from build123d import *

# Parameters (mm, degrees)
BOSS_EXTRUDE1_DEPTH            = 300
CBORE_FOR_M3_SBHCS1_AT_2_COUNT = 2
CBORE_FOR_M3_SBHCS1_AT_2_PITCH = 124.99999999999997
CBORE_FOR_M3_SBHCS1_AT_3_COUNT = 2
CBORE_FOR_M3_SBHCS1_AT_3_PITCH = 249.99999999999997
BOSS_EXTRUDE2_DEPTH            = 5
FILLET1_R                      = 1
LPATTERN1_COUNT                = 2
LPATTERN1_PITCH                = 305
CHAMFER2_SIZE                  = 0.5
FILLET2_R                      = 1


with BuildPart() as part:
    # Sketch1 → Boss-Extrude1 (new body)
    with BuildSketch(Plane.XY):
        Polygon((20, 20), (20, 3.5), (21.600000000000005, 3.5), (24.999999999999996, 7.527677706789349), (25.000000000000004, 11.52767770678935), (40.03508193257454, 17), (44.2305800884609, 12), (45.45625119745129, 13.028460175498461), (45.456251197451294, 20), align=None)
    extrude(amount=BOSS_EXTRUDE1_DEPTH)

    # Sketch4 → CBORE for M3 SBHCS1 (revolve, cut)
    with BuildSketch(Plane(origin=(25, 7.527677706789349, 274.99999999999994), x_dir=(0, 0, -1), z_dir=(2.31e-15, 1, 0))):
        Polygon((0, 0), (-1.22e-15, 5.000000000000024), (1.7999999999999992, 5.000000000000024), (1.8000000000000005, 1.6499999999999997), (3.3499999999999956, 1.6499999999999952), (3.350000000000001, 0.02499999999999889), (3.3749999999999996, -3.47e-15), align=None)
    cbore_for_m3_sbhcs1 = revolve(axis=Axis((31.34999999999999, 7.527677706789334, 274.99999999999994), (-1, 2.32e-15, 0)), mode=Mode.SUBTRACT)

    # CBORE for M3 SBHCS1 at 2: CBORE for M3 SBHCS1 ×2
    with Locations(*[(0, 0, -i * CBORE_FOR_M3_SBHCS1_AT_2_PITCH) for i in range(1, CBORE_FOR_M3_SBHCS1_AT_2_COUNT)]):
        add(cbore_for_m3_sbhcs1, mode=Mode.SUBTRACT)

    # CBORE for M3 SBHCS1 at 3: CBORE for M3 SBHCS1 ×2
    with Locations(*[(0, 0, -i * CBORE_FOR_M3_SBHCS1_AT_3_PITCH) for i in range(1, CBORE_FOR_M3_SBHCS1_AT_3_COUNT)]):
        add(cbore_for_m3_sbhcs1, mode=Mode.SUBTRACT)

    # Sketch5 → Boss-Extrude2 (add)
    with BuildSketch(Plane.XY.offset(300)):
        with BuildLine():
            Line((24.999999999999996, 7.527677706789349), (21.600000000000005, 3.5))
            Line((21.600000000000005, 3.5), (33.71474845278774, 8.05027495743257))
            Line((33.71474845278774, 8.050274957432569), (33.70794748463962, 8.069572384153874))
            Line((33.70794748463962, 8.069572384153874), (32.53600076787437, 11.394915981634217))
            ThreePointArc((32.53600076787437, 11.394915981634217), (32.24344854430553, 11.821955076935874), (31.77657133911045, 12.045505670091789))
            Line((31.77657133911045, 12.045505670091789), (31.704265005172275, 12.059019247038602))
            ThreePointArc((31.704265005172275, 12.0590192470386), (31.23738779997721, 12.282569840194535), (30.94483557640838, 12.70960893549619))
            Line((30.94483557640838, 12.70960893549619), (30.638155724715453, 13.57979856674334))
            Line((30.638155724715453, 13.579798566743342), (25.000000000000004, 11.52767770678935))
            Line((25.000000000000004, 11.52767770678935), (24.999999999999996, 7.527677706789349))
        make_face()
        with BuildLine():
            Line((34.34750801297435, 12.054250698008177), (35.587234405375604, 8.753576884947558))
            Line((35.587234405375604, 8.753576884947558), (44.2305800884609, 12))
            Line((44.2305800884609, 12), (40.03508193257454, 17))
            Line((40.03508193257454, 17), (34.396926207859096, 14.947879140046009))
            Line((34.396926207859096, 14.947879140046007), (34.721342924696536, 14.084145199760654))
            ThreePointArc((34.721342924696536, 14.084145199760654), (34.77173035882119, 13.568965329313977), (34.5577772215813, 13.097612756926463))
            Line((34.5577772215813, 13.097612756926463), (34.511073716089605, 13.04078314084238))
            ThreePointArc((34.511073716089605, 13.04078314084238), (34.297120578849714, 12.569430568454859), (34.34750801297435, 12.054250698008177))
        make_face()
        Polygon((20, 3.5), (21.600000000000005, 3.5), (24.999999999999996, 7.527677706789349), (25.000000000000004, 11.52767770678935), (30.638155724715453, 13.579798566743342), (34.396926207859096, 14.947879140046007), (40.03508193257454, 17), (44.2305800884609, 12), (45.45625119745129, 13.028460175498461), (45.456251197451294, 20), (20, 20), align=None)
    boss_extrude2 = extrude(amount=BOSS_EXTRUDE2_DEPTH)

    # Fillet1
    fillet1_edges = [part.edges().sort_by_distance(p)[0] for p in [
        (35.587234405375604, 8.753576884947558, 302.5),
        (33.71474845278774, 8.05027495743257, 302.5),
    ]]
    fillet(fillet1_edges, radius=FILLET1_R)

    # LPattern1: Boss-Extrude2 ×2
    with Locations(*[(0, 0, -i * LPATTERN1_PITCH) for i in range(1, LPATTERN1_COUNT)]):
        add(boss_extrude2)

    # Chamfer2
    chamfer2_edges = [part.edges().sort_by_distance(p)[0] for p in [
        (33.35225539318084, 8.219308247155407, 300),
        (40.37697975127303, 10.552595526139491, 305),
        (35.758439525002586, 9.13075281507476, 305),
        (33.35225539318084, 8.219308247155407, 305),
        (40.37697975127303, 10.552595526139491, 300),
        (35.758439525002586, 9.13075281507476, 300),
        (34.55913456627782, 14.51601216990333, 0),
        (34.53442546883545, 13.069197948884423, 0),
        (34.96737120917498, 10.403913791477867, 0),
        (39.90890724691825, 10.376788442473778, 0),
        (27.65737422639387, 5.775137478716285, 0),
        (32.24344854430553, 11.821955076935874, 0),
        (31.74041817214136, 12.052262458565195, 0),
        (31.23738779997721, 12.282569840194535, 0),
        (30.791495650561917, 13.144703751119765, 0),
        (32.51754096628727, 14.263838853394676, -5),
        (34.55913456627782, 14.51601216990333, -5),
        (34.77173035882119, 13.56896532931398, 0),
        (34.53442546883545, 13.069197948884423, -5),
        (34.297120578849714, 12.569430568454859, 0),
        (34.96737120917498, 10.403913791477867, -5),
        (39.90890724691825, 10.376788442473778, -5),
        (44.84341564295609, 12.51423008774923, -5),
        (45.45625119745129, 16.51423008774923, -5),
        (32.72812559872565, 20, -5),
        (20, 11.75, -5),
        (20.800000000000004, 3.5, -5),
        (27.65737422639387, 5.775137478716285, -5),
        (33.12537461033105, 9.722595469533394, 0),
        (32.24344854430553, 11.821955076935874, -5),
        (31.74041817214136, 12.052262458565195, -5),
        (31.23738779997721, 12.282569840194535, -5),
        (30.791495650561917, 13.144703751119765, -5),
        (33.12537461033105, 9.722595469533394, -5),
        (34.297120578849714, 12.569430568454859, -5),
        (34.77173035882119, 13.56896532931398, -5),
        (45.456251197451294, 20, 150),
        (20, 3.5, 150),
        (20, 20, 150),
        (30.791495650561917, 13.144703751119765, 300),
        (32.9625451430224, 10.184616411996103, 300),
        (34.297120578849714, 12.569430568454859, 300),
        (34.77173035882119, 13.56896532931398, 300),
        (30.791495650561917, 13.144703751119765, 305),
        (34.55913456627782, 14.51601216990333, 300),
        (34.77173035882119, 13.56896532931398, 305),
        (34.53442546883545, 13.069197948884423, 300),
        (34.297120578849714, 12.569430568454859, 305),
        (34.79156412550927, 10.871986295832649, 300),
        (27.19878088673786, 5.602890750093377, 300),
        (32.9625451430224, 10.184616411996103, 305),
        (32.24344854430553, 11.821955076935874, 300),
        (31.74041817214136, 12.052262458565195, 300),
        (31.23738779997721, 12.282569840194535, 300),
        (32.51754096628727, 14.263838853394676, 305),
        (34.55913456627782, 14.51601216990333, 305),
        (34.53442546883545, 13.069197948884423, 305),
        (34.79156412550927, 10.871986295832649, 305),
        (44.84341564295609, 12.51423008774923, 305),
        (45.45625119745129, 16.51423008774923, 305),
        (32.72812559872565, 20, 305),
        (20, 11.75, 305),
        (20.800000000000004, 3.5, 305),
        (27.19878088673786, 5.602890750093377, 305),
        (32.24344854430553, 11.821955076935874, 305),
        (31.74041817214136, 12.052262458565195, 305),
        (31.23738779997721, 12.282569840194535, 305),
    ]]
    chamfer(chamfer2_edges, length=CHAMFER2_SIZE)

    # Fillet2
    fillet2_edges = [part.edges().sort_by_distance(p)[0] for p in [
        (35.587234405375604, 8.753576884947558, -2.5),
        (33.71474845278774, 8.05027495743257, -2.5),
    ]]
    fillet(fillet2_edges, radius=FILLET2_R)


solid = part.part
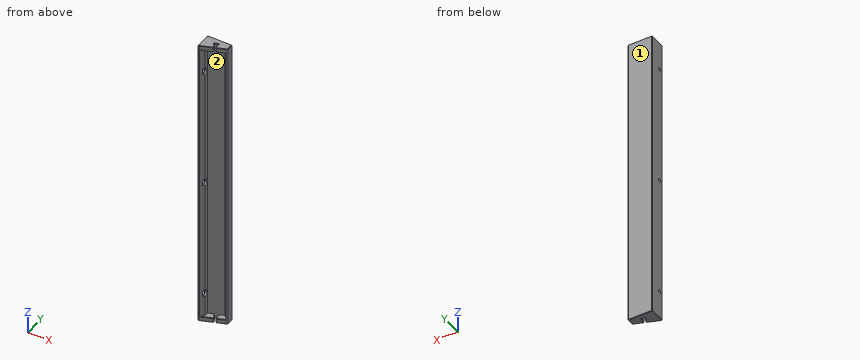
Here's how the part is built. I have some questions about the finished solid (model axes, mm). Face numbers are marked on the shaded views. Coordinates: 2 decimals unless noted, no trailing zeros. Order: outer loops, then holes, each group sorted by start corner. A loop starts at its lowest first (then second) coordinate and runs counter-clockwise, first axis right, second up. Notation, with made-up numbers: M -15.75,75 L 12.25,75 A16 ccw 12.25,103 Z; hole C 21.5,75 d7. An arc over 180 degrees is marked long. Answer as CSV lines item,"result". Start each with the question number.
1. I need wall thicknesses on line 1 (Z direction, x = 38, y = 15); line 2 (X direction, y = 11.5, z = 174); line 3 (Y direction, x = 36, z = 51). Which ranges of each line are inside material? Lowest first, please. Write a range as [from, to].
2. We'd pull the mould along Z, two halves only. Please class the marked faces 1 and 2: released by +Z, released by -Z, zero draft, split by the parting line, or undercut.
3. For pin 1 (6 mm diameter, centred on y = 7.53, z = 150, fed in from +X); pin 2 (2 mm diameter, centred on y = 7.53, z = 275, fed in from +X), each with a flat end and sliding along its axis, tell me the tip position at first contact or that it passes through.
4. I want a section at A-A, the plane z = 117.5. Write out the boundary of the cut face in (x, y).
Recorded:
1,line 1,"z = [-5, 0], [300, 305]"
1,line 2,"x = [20, 25]"
1,line 3,"y = [15.53, 20]"
2,face 1,"zero draft"
2,face 2,"undercut"
3,pin 1,"stops at x = 23.35"
3,pin 2,"passes through"
4,outline,"M 20,4 L 20.5,3.5 L 21.6,3.5 L 25,7.53 L 25,11.53 L 40.04,17 L 44.23,12 L 45.46,13.03 L 45.46,19.5 L 44.96,20 L 20.5,20 L 20,19.5 Z"
